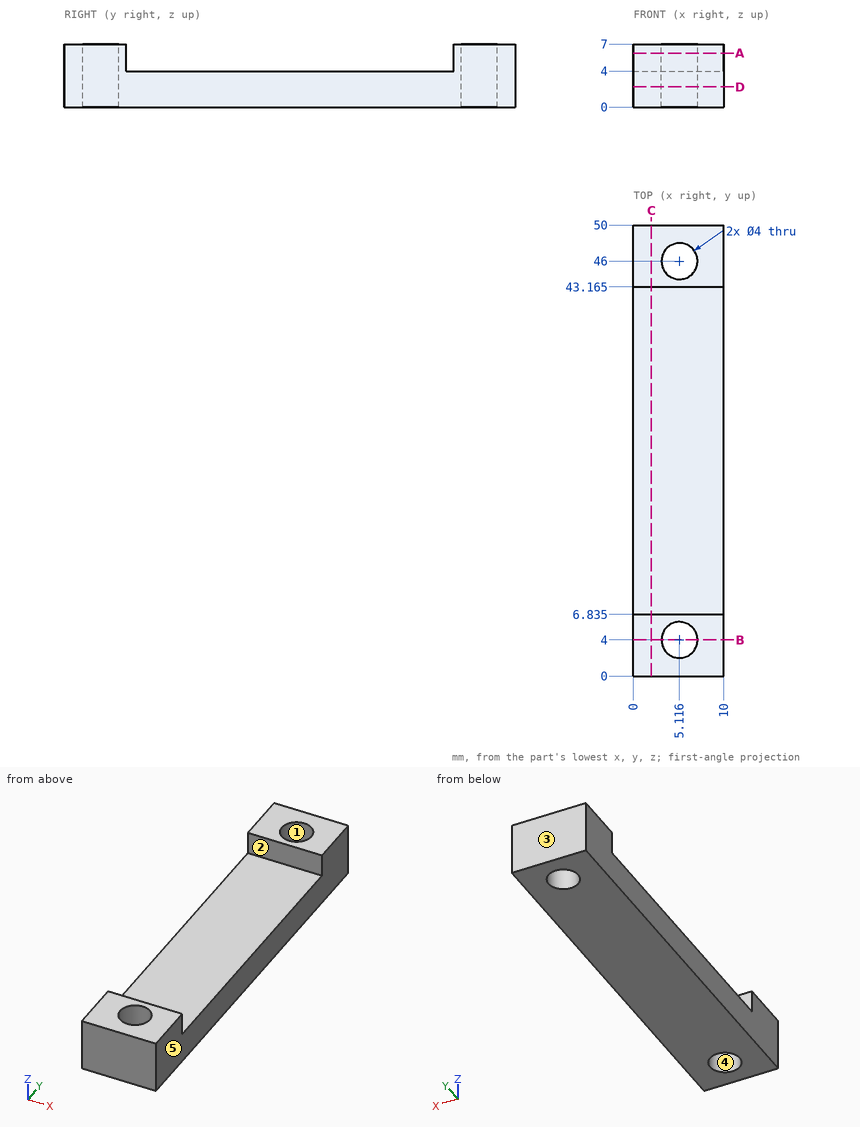
Job drawing, mm, ordinate dimensions from the low corner. One solid piece. A direction names the side the tool comes from. Give positions to 0.01 mm unless a question says otherwise; leave off trailing zeros. Loops run counter-clockwise (first coordinate to the right, second up) from the corner with the lowest first, then second, coordinate; pieces in that order, holes last. Notation, with made-up numbers: M 43.25,59 L 48.25,59 A17 ccw 48.25,69 Z; hole C -7,2.25 d2. An arc over 180 degrees is marked long. Return JSON: item names as keys, results as strings.
1) 3-axis set-ups, long thin cutter, end or side, ignore diameter. For the marked faces 1 and 2: which of +Z, -Z, +X, -X, +Y, -Y reach the whole face in a straight line?
Calculated:
{"face 1": "+Z, -Z", "face 2": "+Z, +X, -X"}
2) Saw through at C-C, the plane x = 2. List the corners of the cut face in (y, z) (1 decimal).
Calculated:
{"outline": "M 0,0 L 50,0 L 50,7 L 43.2,7 L 43.2,4 L 6.8,4 L 6.8,7 L 0,7 Z"}
3) Drill centre lines: line 1 (Y direction, x = 8, z = 6.5) (1 decimal); line 2 (X direction, y = 4, z = 3); line 3 (Y direction, x = 4.5, z = 3.25). Where is each one in solid material? Low to high.
Calculated:
{"line 1": "y = 0 to 6.8, 43.2 to 50", "line 2": "x = 0 to 3.12, 7.12 to 10", "line 3": "y = 0 to 2.1, 5.9 to 44.1, 47.9 to 50"}
4) Saw through at A-A, the plane z = 6. List the corners of the cut face in (x, y) (1 decimal).
Calculated:
{"outline": "M 0,0 L 10,0 L 10,6.8 L 0,6.8 Z; M 0,43.2 L 10,43.2 L 10,50 L 0,50 Z; hole C 5.1,4 d4; hole C 5.1,46 d4"}
5) Flat gauge pins, fed straight in: pin 1 Ø3 at (x, y) = (4.5, 26) entering from +Z; pin 2 Ø2.5 at (x, y) = (5.12, 4) entering from +Z. Where does each tip first touch, or does it go through?
Calculated:
{"pin 1": "stops at z = 4", "pin 2": "passes through"}
6) Saw through at D-D, the plane z = 2.25. List the corners of the cut face in (x, y), then the cut area to 3 significant figures.
Calculated:
{"outline": "M 0,0 L 10,0 L 10,50 L 0,50 Z; hole C 5.12,4 d4; hole C 5.12,46 d4", "area": "475 mm2"}
7) Saw through at B-B, the plane y = 4. List the corners of the cut face in (x, z), then the cut area to 3 significant figures.
Calculated:
{"outline": "M 0,0 L 3.12,0 L 3.12,7 L 0,7 Z; M 7.12,0 L 10,0 L 10,7 L 7.12,7 Z", "area": "42.0 mm2"}
8) Pull direction X, two halves, no side cores. Call the marked faces 3, 4 and 5: released by +X, released by -X, zero draft, split by the parting line, or undercut.
Calculated:
{"face 3": "zero draft", "face 4": "undercut", "face 5": "released by +X"}
